```python
from build123d import *

# Parameters (mm, degrees)
SKETCH1_R           = 2.25
SKETCH1_R_2         = 5
SKETCH1_R_3         = 0.75
SKETCH1_R_4         = 0.875
BOSS_EXTRUDE1_DEPTH = 1


with BuildPart() as part:
    # Sketch1 → Boss-Extrude1 (new body)
    with BuildSketch(Plane.XY):
        Polygon((-25, 25), (-25, -25), (-5.5, -25), (-5.5, -7.5), (5.5, -7.5), (5.5, -25), (25, -25), (25, 25), align=None)
        with Locations((-15, -15)):
            Circle(SKETCH1_R, mode=Mode.SUBTRACT)
        Circle(SKETCH1_R_2, mode=Mode.SUBTRACT)
        with Locations((15, -15)):
            Circle(SKETCH1_R, mode=Mode.SUBTRACT)
        with Locations((-9.8, 0)):
            Circle(SKETCH1_R_3, mode=Mode.SUBTRACT)
        with Locations((-7, 0)):
            Circle(SKETCH1_R_4, mode=Mode.SUBTRACT)
        with Locations((-15, 15)):
            Circle(SKETCH1_R, mode=Mode.SUBTRACT)
        with Locations((7, 0)):
            Circle(SKETCH1_R_4, mode=Mode.SUBTRACT)
        with Locations((9.8, 0)):
            Circle(SKETCH1_R_3, mode=Mode.SUBTRACT)
        with Locations((15, 15)):
            Circle(SKETCH1_R, mode=Mode.SUBTRACT)
    extrude(amount=BOSS_EXTRUDE1_DEPTH)


solid = part.part
```
Geometry check sheet. Reference: the model listing, model coordinates, mm. Round coordinates to 2 decimals unless told otherwise and drop trailing zeros. Order: outer loops, then holes, each group sorted by start corner. A loop starts at its lowest first (then second) coordinate and runs counter-clockwise, first axis right, second up. Notation, with made-up numbers: (-0.5, 77.25) -> (49.5, 77.25) arc R11 ccw to (49.5, 94.25) -> close; hole circle Ø2 at (20.5, 17.25). An arc over 180 degrees is marked (long way). Return JSON: item names as keys, results as strings. Group by question number.
Q1. Material ranges on probe 1 along Y at (x, z) = (-15, 0.75); probe 2 along Y at (x, z) = (0, 0.1); probe 3 along Y at (x, z) = (-13.5, 0.45), recorded low to high. Write a range as from..to.
Q2. Section check B-B, the plane x = 0. Record the boundary of the cut face in (y, z).
Q3. Release check for a two-part mould opening along Y. For faces 1 (the cylindrical face through (-9.085, 0.225, 0.493)), 2 (the cylindrical face through (-6.165, 0.263, 0.493)), 3 (the flat face through (0, 6, 0)) record: released by +Y, released by -Y, zero draft, split by the parting line, or undercut.
Q4. Section check C-C, the plane y = -21. Record the boundary of the cut face in (x, z), plus the area to 3 significant figures.
Q5. Section check D-D, the plane y = 0. Record the boundary of the cut face in (x, z) (3 decimals), plus the area to 3 significant figures.
Q6. Gauge pin test, flat end, axial feed: pin 1 (9 mm diameter, centred on x = 0, y = 0, fed in from +Z). Record the tip position at first contact, or that the pin passes through.
Q7. Section check A-A, the plane y = 15. Record the boundary of the cut face in (x, z), plus the area to 3 significant figures.
Numbers:
{
 "1": {"probe 1": "-25..-17.25, -12.75..12.75, 17.25..25", "probe 2": "-7.5..-5, 5..25", "probe 3": "-25..-16.68, -13.32..13.32, 16.68..25"},
 "2": {"outline": "(-7.5, 0) -> (-5, 0) -> (-5, 1) -> (-7.5, 1) -> close; (5, 0) -> (25, 0) -> (25, 1) -> (5, 1) -> close"},
 "3": {"face 1": "undercut", "face 2": "undercut", "face 3": "zero draft"},
 "4": {"outline": "(-25, 0) -> (-5.5, 0) -> (-5.5, 1) -> (-25, 1) -> close; (5.5, 0) -> (25, 0) -> (25, 1) -> (5.5, 1) -> close", "area": "39.0 mm^2"},
 "5": {"outline": "(-25, 0) -> (-10.55, 0) -> (-10.55, 1) -> (-25, 1) -> close; (-9.05, 0) -> (-7.875, 0) -> (-7.875, 1) -> (-9.05, 1) -> close; (-6.125, 0) -> (-5, 0) -> (-5, 1) -> (-6.125, 1) -> close; (5, 0) -> (6.125, 0) -> (6.125, 1) -> (5, 1) -> close; (7.875, 0) -> (9.05, 0) -> (9.05, 1) -> (7.875, 1) -> close; (10.55, 0) -> (25, 0) -> (25, 1) -> (10.55, 1) -> close", "area": "33.5 mm^2"},
 "6": {"pin 1": "through"},
 "7": {"outline": "(-25, 0) -> (-17.25, 0) -> (-17.25, 1) -> (-25, 1) -> close; (-12.75, 0) -> (12.75, 0) -> (12.75, 1) -> (-12.75, 1) -> close; (17.25, 0) -> (25, 0) -> (25, 1) -> (17.25, 1) -> close", "area": "41.0 mm^2"}
}
